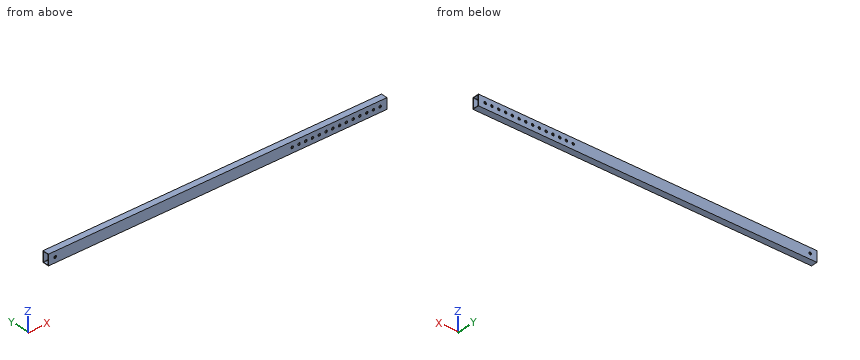
from build123d import *

# Parameters (mm, degrees)
F0_W     = 38.1
F0_H     = 63.5
F1_DEPTH = 2000
F2_R     = 7.5
F3_DEPTH = 38.1
F5_DEPTH = 38.1


with BuildPart() as f1:
    # F0 (on Right) → F1 (new body)
    with BuildSketch(Plane.YZ):
        Rectangle(F0_W, F0_H)
        with BuildLine():
            Line((-14.55, 29.25), (14.55, 29.25))
            ThreePointArc((14.55, 29.25), (15.964214, 28.664214), (16.55, 27.25))
            Line((16.55, 27.25), (16.55, -27.25))
            ThreePointArc((16.55, -27.25), (15.964214, -28.664214), (14.55, -29.25))
            Line((14.55, -29.25), (-14.55, -29.25))
            ThreePointArc((-14.55, -29.25), (-15.964214, -28.664214), (-16.55, -27.25))
            Line((-16.55, -27.25), (-16.55, 27.25))
            ThreePointArc((-16.55, 27.25), (-15.964214, 28.664214), (-14.55, 29.25))
        make_face(mode=Mode.SUBTRACT)
    extrude(amount=F1_DEPTH)

    # F2 (on face) → F3 (cut, through all)
    with BuildSketch(Plane.XZ.offset(19.05)):
        with Locations((40, 0)):
            Circle(F2_R)
    extrude(amount=-F3_DEPTH, mode=Mode.SUBTRACT)

    # F4 (on face) → F5 (cut, through all)
    with BuildSketch(Plane.XZ.offset(19.05)):
        with BuildLine():
            Line((1952.5, 0), (1967.5, 0))
            ThreePointArc((1967.5, 0), (1960, 7.5), (1952.5, 0))
        make_face()
        with BuildLine():
            ThreePointArc((1432.5, 0), (1440, -7.5), (1447.5, 0))
            Line((1447.5, 0), (1432.5, 0))
        make_face()
        with BuildLine():
            Line((1432.5, 0), (1447.5, 0))
            ThreePointArc((1447.5, 0), (1440, 7.5), (1432.5, 0))
        make_face()
        with BuildLine():
            ThreePointArc((1472.5, 0), (1480, -7.5), (1487.5, 0))
            Line((1487.5, 0), (1472.5, 0))
        make_face()
        with BuildLine():
            Line((1472.5, 0), (1487.5, 0))
            ThreePointArc((1487.5, 0), (1480, 7.5), (1472.5, 0))
        make_face()
        with BuildLine():
            ThreePointArc((1512.5, 0), (1520, -7.5), (1527.5, 0))
            Line((1527.5, 0), (1512.5, 0))
        make_face()
        with BuildLine():
            Line((1512.5, 0), (1527.5, 0))
            ThreePointArc((1527.5, 0), (1520, 7.5), (1512.5, 0))
        make_face()
        with BuildLine():
            ThreePointArc((1552.5, 0), (1560, -7.5), (1567.5, 0))
            Line((1567.5, 0), (1552.5, 0))
        make_face()
        with BuildLine():
            Line((1552.5, 0), (1567.5, 0))
            ThreePointArc((1567.5, 0), (1560, 7.5), (1552.5, 0))
        make_face()
        with BuildLine():
            ThreePointArc((1592.5, 0), (1600, -7.5), (1607.5, 0))
            Line((1607.5, 0), (1592.5, 0))
        make_face()
        with BuildLine():
            Line((1592.5, 0), (1607.5, 0))
            ThreePointArc((1607.5, 0), (1600, 7.5), (1592.5, 0))
        make_face()
        with BuildLine():
            ThreePointArc((1632.5, 0), (1640, -7.5), (1647.5, 0))
            Line((1647.5, 0), (1632.5, 0))
        make_face()
        with BuildLine():
            Line((1632.5, 0), (1647.5, 0))
            ThreePointArc((1647.5, 0), (1640, 7.5), (1632.5, 0))
        make_face()
        with BuildLine():
            ThreePointArc((1672.5, 0), (1680, -7.5), (1687.5, 0))
            Line((1687.5, 0), (1672.5, 0))
        make_face()
        with BuildLine():
            Line((1672.5, 0), (1687.5, 0))
            ThreePointArc((1687.5, 0), (1680, 7.5), (1672.5, 0))
        make_face()
        with BuildLine():
            ThreePointArc((1712.5, 0), (1720, -7.5), (1727.5, 0))
            Line((1727.5, 0), (1712.5, 0))
        make_face()
        with BuildLine():
            Line((1712.5, 0), (1727.5, 0))
            ThreePointArc((1727.5, 0), (1720, 7.5), (1712.5, 0))
        make_face()
        with BuildLine():
            ThreePointArc((1752.5, 0), (1760, -7.5), (1767.5, 0))
            Line((1767.5, 0), (1752.5, 0))
        make_face()
        with BuildLine():
            Line((1752.5, 0), (1767.5, 0))
            ThreePointArc((1767.5, 0), (1760, 7.5), (1752.5, 0))
        make_face()
        with BuildLine():
            ThreePointArc((1792.5, 0), (1800, -7.5), (1807.5, 0))
            Line((1807.5, 0), (1792.5, 0))
        make_face()
        with BuildLine():
            Line((1792.5, 0), (1807.5, 0))
            ThreePointArc((1807.5, 0), (1800, 7.5), (1792.5, 0))
        make_face()
        with BuildLine():
            ThreePointArc((1832.5, 0), (1840, -7.5), (1847.5, 0))
            Line((1847.5, 0), (1832.5, 0))
        make_face()
        with BuildLine():
            Line((1832.5, 0), (1847.5, 0))
            ThreePointArc((1847.5, 0), (1840, 7.5), (1832.5, 0))
        make_face()
        with BuildLine():
            ThreePointArc((1872.5, 0), (1880, -7.5), (1887.5, 0))
            Line((1887.5, 0), (1872.5, 0))
        make_face()
        with BuildLine():
            Line((1872.5, 0), (1887.5, 0))
            ThreePointArc((1887.5, 0), (1880, 7.5), (1872.5, 0))
        make_face()
        with BuildLine():
            ThreePointArc((1912.5, 0), (1920, -7.5), (1927.5, 0))
            Line((1927.5, 0), (1912.5, 0))
        make_face()
        with BuildLine():
            Line((1912.5, 0), (1927.5, 0))
            ThreePointArc((1927.5, 0), (1920, 7.5), (1912.5, 0))
        make_face()
        with BuildLine():
            ThreePointArc((1952.5, 0), (1960, -7.5), (1967.5, 0))
            Line((1967.5, 0), (1952.5, 0))
        make_face()
    extrude(amount=-F5_DEPTH, mode=Mode.SUBTRACT)


solid = f1.part
Verification items for the finished model (mm, model axes). Coordinates: 2 decimals unless noted, no trailing zeros. Write each loop counter-clockwise with the first axis right and the second up, starting at its lowest first coordinate (ties: lowest second). Pieces come first, ordered by that corner, then holes. Notation, with made-up numbers: (26, 48) -> (45, 48) arc R37 ccw to (45, 84) -> close; hole circle Ø3 at (39, -32.5). An arc over 180 degrees is marked (long way). One line per item, written item: value. Start each with the question number.
Q1. Go/stop test with a flat-tipped pin: P1, Ø17, axis at x = 40, z = 0, coming from the +Y side. Record where the tip stops, or that it passes through.
Q2. Cross-section at B-B on y = -7.5. Enter the section's corners in (x, z).
Q3. Thickness scan on L1, parallel to Z at x = 856, y = -14; L2, parallel to Y at x = 396.5, z = 3; L3, parallel to Z at x = 99, y = -15.5. Record the ranges inside material, lowest first. Write a range as from..to.
Q4. Cross-section at A-A on x = 687. Enter the section's corners in (y, z).
Checked values:
1. P1: stops at y = 19.05
2. outline: (0, -31.75) -> (2000, -31.75) -> (2000, -29.25) -> (0, -29.25) -> close; (0, 29.25) -> (2000, 29.25) -> (2000, 31.75) -> (0, 31.75) -> close
3. L1: z = -31.75..-29.25, 29.25..31.75
3. L2: y = -19.05..-16.55, 16.55..19.05
3. L3: z = -31.75..-29.01, 29.01..31.75
4. outline: (-19.05, -31.75) -> (19.05, -31.75) -> (19.05, 31.75) -> (-19.05, 31.75) -> close; hole (-16.55, -27.25) arc R2 ccw to (-14.55, -29.25) -> (14.55, -29.25) arc R2 ccw to (16.55, -27.25) -> (16.55, 27.25) arc R2 ccw to (14.55, 29.25) -> (-14.55, 29.25) arc R2 ccw to (-16.55, 27.25) -> close
